from build123d import *

# Parameters (mm, degrees)
SKETCH_2_W      = 23
SKETCH_2_H      = 23
SKETCH_2_R      = 1.75
EXTRUDE_1_DEPTH = 1.7
SKETCH_2_3_W    = 3
SKETCH_2_3_H    = 5
EXTRUDE_2_DEPTH = 3.1
FILLET_2_R      = 4.25
FILLET_3_R      = 4.25
FILLET_4_R      = 4.25
FILLET_5_R      = 4.25
FILLET_6_R      = 0.5


with BuildPart() as part:
    # 草图2 → 凸台-拉伸1 (new body)
    with BuildSketch(Plane.XY):
        Rectangle(SKETCH_2_W, SKETCH_2_H)
        with Locations((8, 8)):
            Circle(SKETCH_2_R, mode=Mode.SUBTRACT)
        with Locations((-8, 8)):
            Circle(SKETCH_2_R, mode=Mode.SUBTRACT)
        with Locations((8, -8)):
            Circle(SKETCH_2_R, mode=Mode.SUBTRACT)
        with Locations((-8, -8)):
            Circle(SKETCH_2_R, mode=Mode.SUBTRACT)
    extrude(amount=EXTRUDE_1_DEPTH)

    # 草图2<3> → 凸台-拉伸2 (add)
    with BuildSketch(Plane.XY):
        Rectangle(SKETCH_2_3_W, SKETCH_2_3_H)
    extrude(amount=EXTRUDE_2_DEPTH)

    # 圆角2
    fillet_2_edges = [part.edges().sort_by_distance(p)[0] for p in [
        (11.5, 11.5, 0.85),
    ]]
    fillet(fillet_2_edges, radius=FILLET_2_R)

    # 圆角3
    fillet_3_edges = [part.edges().sort_by_distance(p)[0] for p in [
        (-11.5, 11.5, 0.85),
    ]]
    fillet(fillet_3_edges, radius=FILLET_3_R)

    # 圆角4
    fillet_4_edges = [part.edges().sort_by_distance(p)[0] for p in [
        (-11.5, -11.5, 0.85),
    ]]
    fillet(fillet_4_edges, radius=FILLET_4_R)

    # 圆角5
    fillet_5_edges = [part.edges().sort_by_distance(p)[0] for p in [
        (11.5, -11.5, 0.85),
    ]]
    fillet(fillet_5_edges, radius=FILLET_5_R)

    # 圆角6
    fillet_6_edges = [part.edges().sort_by_distance(p)[0] for p in [
        (0, 2.5, 3.1),
        (1.5, 0, 3.1),
        (-1.5, 0, 3.1),
        (0, -2.5, 3.1),
    ]]
    fillet(fillet_6_edges, radius=FILLET_6_R)


solid = part.part
Work out the finished part from the listing and answer in its coordinate system (mm). A direction names the side the tool comes from. Round coordinates to 2 decimals unless told otherwise and drop trailing zeros. Loops run counter-clockwise (first coordinate to the right, second up) from the corner with the lowest first, then second, coordinate; pieces in that order, holes last. Notation, with made-up numbers: (20.5, -9) -> (47.5, -9) arc R9 ccw to (47.5, 0) -> close; hole circle Ø1 at (-35.75, -6). An arc over 180 degrees is marked (long way). Use one line per item in the form item = value.
(1) A tool of negligible diameter and unlimited length cuts with its end or side. For faces 1 (the flat face through (0, 2.5, 2)), 2 (the flat face through (1.5, 0, 2)), 3 (the flat face through (-1.5, 0, 2)), from which of +Z, -Z, +X, -X, +Y, -Y can it reach the whole face along a straight path? Write none if from no direction.
Answer list:
face_1 = +Z, +X, -X, +Y
face_2 = +Z, +X, +Y, -Y
face_3 = +Z, -X, +Y, -Y
(2) Straight lines are drawn through the part: line 1 (Y direction, x = -8, z = 0.7); line 2 (X direction, y = -8.25, z = 1.1); line 3 (Z direction, x = -8.75, y = -3). For each, find the intervals that lie inside material, in ascending order.
Answer list:
line_1 = -11.43 to -9.75, -6.25 to 6.25, 9.75 to 11.43
line_2 = -11.38 to -9.73, -6.27 to 6.27, 9.73 to 11.38
line_3 = 0 to 1.7
(3) Find section A-A on z = 1.3. Give the vertices of the cut face in (x, y), then the cut area to 3 significant figures.
Answer list:
outline = (-11.5, -7.25) arc R4.25 ccw to (-7.25, -11.5) -> (7.25, -11.5) arc R4.25 ccw to (11.5, -7.25) -> (11.5, 7.25) arc R4.25 ccw to (7.25, 11.5) -> (-7.25, 11.5) arc R4.25 ccw to (-11.5, 7.25) -> close; hole circle Ø3.5 at (-8, -8); hole circle Ø3.5 at (-8, 8); hole circle Ø3.5 at (8, -8); hole circle Ø3.5 at (8, 8)
area = 475 mm2
(4) Find section D-D on x = 4. Give the vertices of the cut face in (y, z).
Answer list:
outline = (-11.5, 0) -> (11.5, 0) -> (11.5, 1.7) -> (-11.5, 1.7) -> close
(5) Find section B-B on x = 8. Give the vertices of the cut face in (y, z), then the cut area to 3 significant figures.
Answer list:
outline = (-11.43, 0) -> (-9.75, 0) -> (-9.75, 1.7) -> (-11.43, 1.7) -> close; (-6.25, 0) -> (6.25, 0) -> (6.25, 1.7) -> (-6.25, 1.7) -> close; (9.75, 0) -> (11.43, 0) -> (11.43, 1.7) -> (9.75, 1.7) -> close
area = 27.0 mm2
(6) For a pull along X with two mould halves and no side action, classify faces 4 (the cylindrical face through (-10.22, 10.29, 0.86)), 5 (the flat face through (11.5, 0, 1)), 6 (the cylindrical face through (9.669, 8.526, 0.838)), 7 (the flat face through (0, 0, 3.1)) as released by +X, released by -X, zero draft, split by the parting line, or undercut.
Answer list:
face_4 = released by -X
face_5 = released by +X
face_6 = undercut
face_7 = zero draft
